Can you work these out from the model? Positions are in its coordinate system, mm. A direction names the side the tool comes from. Coordinates: 2 decimals unless noted, no trailing zeros. Write each loop counter-clockwise with the first axis right and the second up, starting at its lowest first coordinate (ties: lowest second). Pieces come first, ordered by that corner, then holes. Notation, with made-up numbers: M 72,83 L 97,83 A32 ccw 97,119 Z; hole C 16,85 d7. An arc over 180 degrees is marked long. Use one line per item in the form item = value. Start each with the question number.
```python
from build123d import *

# Parameters (mm, degrees)
SKETCH1_W           = 5
SKETCH1_H           = 15
BOSS_EXTRUDE1_DEPTH = 5
SKETCH4_W           = 3
SKETCH4_H           = 8
CUT_EXTRUDE3_DEPTH  = 15
SKETCH5_W           = 6
SKETCH5_H           = 4
CUT_EXTRUDE5_DEPTH  = 2


with BuildPart() as part:
    # Sketch1 → Boss-Extrude1 (new, symmetric)
    with BuildSketch(Plane.XY):
        Rectangle(SKETCH1_W, SKETCH1_H)
    extrude(amount=BOSS_EXTRUDE1_DEPTH, both=True)

    # Sketch4 → Cut-Extrude3 (cut)
    with BuildSketch(Plane(origin=(0, 7.5, 0), x_dir=(1, 0, 0), z_dir=(0, 1, 0))):
        with Locations((-1, 1)):
            Rectangle(SKETCH4_W, SKETCH4_H)
    extrude(amount=-CUT_EXTRUDE3_DEPTH, mode=Mode.SUBTRACT)

    # Sketch5 → Cut-Extrude5 (cut)
    with BuildSketch(Plane.ZY.offset(-0.5)):
        Rectangle(SKETCH5_W, SKETCH5_H)
    extrude(amount=-CUT_EXTRUDE5_DEPTH, mode=Mode.SUBTRACT)


solid = part.part
```
1) Suppose I cut it at D-D on y = 4.5. Please give me the cut outline in (x, z).
2) Suppose I cut it at C-C on x = 1. Please give me the cut outline in (y, z).
3) Please list where these lines run through material, in increasing order: line 1 (Y direction, x = 1.1, z = -2); line 2 (Z direction, x = 1.15, y = 1); line 3 (X direction, y = -3.25, z = -2.75).
4) Suppose I cut it at A-A on y = -0.5. Please give me the cut outline in (x, z).
5) Suppose I cut it at B-B on z = 0.5. Please give me the cut outline in (x, y).
6) Which directions (+Z, -Z, +X, -X, +Y, -Y) give clear straight access to the entire face, cutting with the end or side of a thin tool? Please do faces 5 (the face through (-1, 0, 3)), 6 (the face through (1, 0, -3)), 7 (the face through (0.5, 0, -4)).
7) Will these pins go through, and if not, where does the flat tip stop? pin 1 Ø5 at (y, z) = (-1.5, 1.5) entering from +X; pin 2 Ø2.5 at (y, z) = (3, -2.5) entering from -X.
8) If we mould it in two halves opening along Z, with no side actions, what happens to faces 1 (the face through (1, 7.5, 1)), 2 (the face through (1, -2, 0)), 3 (the face through (1, 0, -5)), 4 (the face through (1, 2, 0))? For each: +Z half, -Z half, draft (parallel to the pull), parting line (faces both ways), or undercut.
Computed values:
q1.outline = M -2.5,3 L 0.5,3 L 0.5,-5 L 2.5,-5 L 2.5,5 L -2.5,5 Z
q2.outline = M -7.5,-5 L 7.5,-5 L 7.5,5 L -7.5,5 Z; hole M -2,-3 L 2,-3 L 2,3 L -2,3 Z
q3.line_1 = -7.5 to -2, 2 to 7.5
q3.line_2 = -5 to -3, 3 to 5
q3.line_3 = 0.5 to 2.5
q4.outline = M -2.5,3 L 2.5,3 L 2.5,5 L -2.5,5 Z; M 0.5,-5 L 2.5,-5 L 2.5,-3 L 0.5,-3 Z
q5.outline = M 0.5,-7.5 L 2.5,-7.5 L 2.5,-2 L 0.5,-2 Z; M 0.5,2 L 2.5,2 L 2.5,7.5 L 0.5,7.5 Z
q6.face_5 = -X
q6.face_6 = +X, -X
q6.face_7 = -Z, -X, +Y, -Y
q7.pin_1 = 2.5
q7.pin_2 = 0.5
q8.face_1 = draft
q8.face_2 = undercut
q8.face_3 = -Z half
q8.face_4 = undercut
